Geometry check sheet. Reference: the model listing, model coordinates, mm. Face numbers are marked on the shaded views. A direction names the side the tool comes from. Give positions to 0.01 mm unless a question says otherwise; leave off trailing zeros. Write each loop counter-clockwise with the first axis right and the second up, starting at its lowest first coordinate (ties: lowest second). Pieces come first, ordered by that corner, then holes. Notation, with made-up numbers: (-19.75, 87) -> (6.25, 87) arc R15 cw to (6.25, 94) -> close; hole circle Ø1 at (-22, 12). An arc over 180 degrees is marked (long way). One line per item, written item: value.
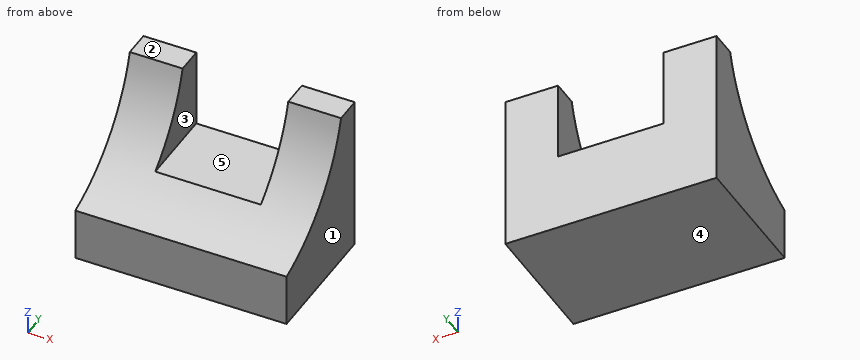
from build123d import *

# Parameters (mm, degrees)
F0_W     = 50.8
F0_H     = 38.1
F1_DEPTH = 31.75
F2_W     = 25.4
F2_H     = 19.05
F3_DEPTH = 38.1
F5_DEPTH = 76.2


with BuildPart() as f1:
    # F0 (on Front) → F1 (new body)
    with BuildSketch(Plane.XZ):
        with Locations((25.4, 19.05)):
            Rectangle(F0_W, F0_H)
    extrude(amount=F1_DEPTH)

    # F2 (on face) → F3 (cut)
    with BuildSketch(Plane.XZ.offset(31.75)):
        with Locations((25.4, 28.575)):
            Rectangle(F2_W, F2_H)
    extrude(amount=-F3_DEPTH, mode=Mode.SUBTRACT)

    # F4 (on face) → F5 (cut)
    with BuildSketch(Plane.YZ.offset(50.8)):
        with BuildLine():
            Line((-6.35, 38.1), (-31.75, 38.1))
            Line((-31.75, 38.1), (-31.75, 12.7))
            ThreePointArc((-31.75, 12.7), (-15.700044, 22.050044), (-6.35, 38.1))
        make_face()
    extrude(amount=-F5_DEPTH, mode=Mode.SUBTRACT)


solid = f1.part
1) Depth check by flat-ended pin: pin 1 Ø15.5 at (x, y) = (26, -10.5) entering from +Z; pin 2 Ø5 at (x, z) = (14, 17.5) entering from -Y. Enter the tip coordinate at first touch or a pass-through.
Verdict:
pin 1: z = 19.05
pin 2: y = -25.63
2) Sectioned sample at D-D on z = 20.5. Record the cut outline in (x, y), plus the area to 3 significant figures.
Verdict:
outline: (0, -17.35) -> (12.7, -17.35) -> (12.7, 0) -> (0, 0) -> close; (38.1, -17.35) -> (50.8, -17.35) -> (50.8, 0) -> (38.1, 0) -> close
area: 441 mm^2
3) Sectioned sample at A-A on z = 25. Record the cut outline in (x, y).
Verdict:
outline: (0, -13.05) -> (12.7, -13.05) -> (12.7, 0) -> (0, 0) -> close; (38.1, -13.05) -> (50.8, -13.05) -> (50.8, 0) -> (38.1, 0) -> close
4) Mould release check, pull along X, two halves, no side actions. Record for the marked faces 1, 2 and 3: released by +X, released by -X, zero draft, split by the parting line, or undercut.
Verdict:
face 1: released by +X
face 2: zero draft
face 3: undercut
5) Sectioned sample at B-B on y = -1.5. Record the cut outline in (x, z).
Verdict:
outline: (0, 0) -> (50.8, 0) -> (50.8, 38.1) -> (38.1, 38.1) -> (38.1, 19.05) -> (12.7, 19.05) -> (12.7, 38.1) -> (0, 38.1) -> close
6) Tool access check on the marked faces 4 and 5. Record the directions out of +Z, -Z, +X, -X, +Y, -Y that give a thin tool (end or side, any length) a straight path to the whole face; none if there is none.
Verdict:
face 4: -Z, +X, -X, +Y, -Y
face 5: +Z, +Y, -Y
7) Sectioned sample at C-C on x = 22. Record the cut outline in (y, z).
Verdict:
outline: (-31.75, 0) -> (0, 0) -> (0, 19.05) -> (-19.1, 19.05) arc R36.41 cw to (-31.75, 12.7) -> close
8) Scan lines: probe 1 along Z at (x, y) = (33.5, -6); probe 2 along Z at (x, y) = (29, -20.5); probe 3 along Y at (x, z) = (27, 16.5). Record each from-to range of solid material in increasing order.
Verdict:
probe 1: 0 to 19.05
probe 2: 0 to 18.01
probe 3: -22.84 to 0
